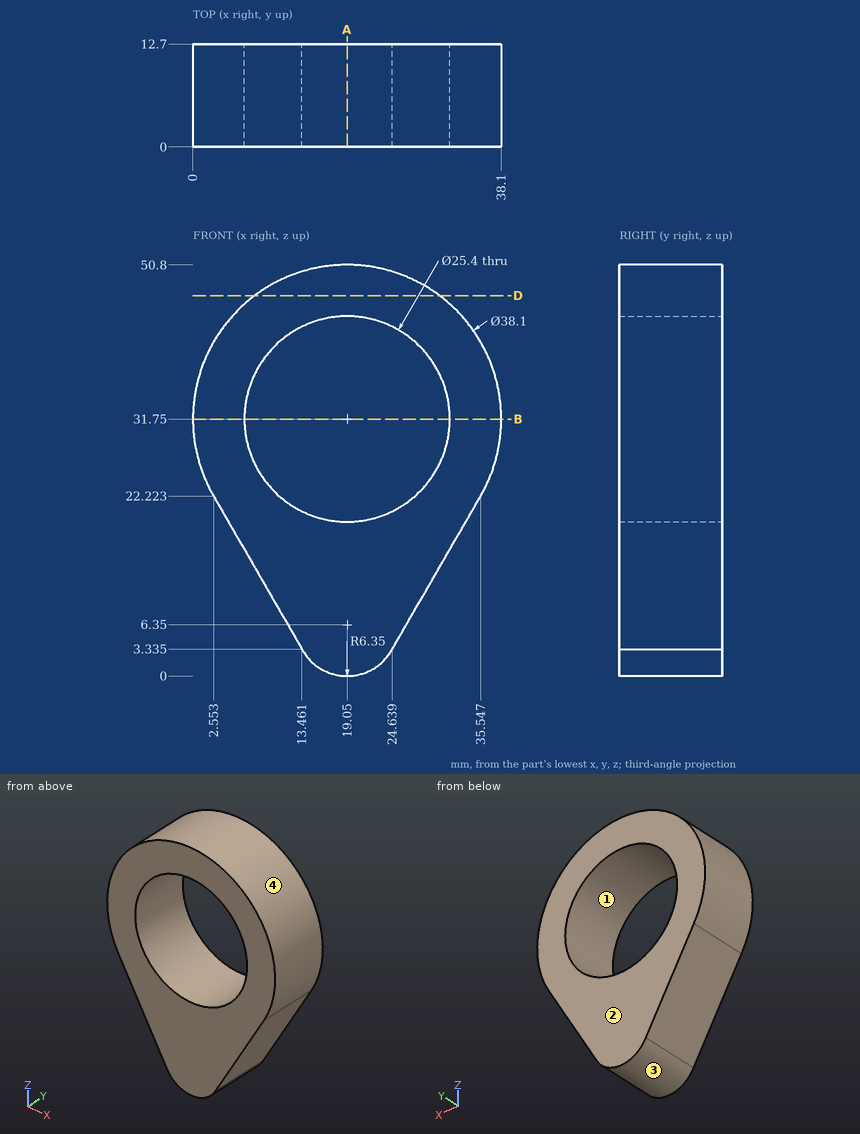
Print and shaded views of the part. All mm, measured from the part's lowest x, y and z. Coordinates: 2 decimals unless noted, no trailing zeros. Order: outer loops, then holes, each group sorted by start corner. A loop starts at its lowest first (then second) coordinate and runs counter-clockwise, first axis right, second up.
Item 1: Saw through at B-B on z = 31.75. List the corners of the cut face in (x, y).
Filled in:
outline: (0, 0) - (6.35, 0) - (6.35, 12.7) - (0, 12.7) - close; (31.75, 0) - (38.1, 0) - (38.1, 12.7) - (31.75, 12.7) - close
Item 2: Drop flat-ended pins along their axis: pin 1 Ø1 at (y, z) = (11, 38) entering from -X; pin 2 Ø5 at (x, y) = (22.5, 3.5) entering from +Z; pin 3 Ø5 at (x, y) = (5, 10) entering from +Z. Give the stop position or say it passes through.
Filled in:
pin 1: stops at x = 0.89
pin 2: stops at z = 50.78
pin 3: stops at z = 46.9
Item 3: Mould opens along Z. For the marked faces 1, 2, 3 and 4 say: released by +Z, released by -Z, zero draft, split by the parting line, or undercut.
Filled in:
face 1: undercut
face 2: zero draft
face 3: released by -Z
face 4: split by the parting line
Item 4: Drill centre lines: L1, parallel to Z at x = 19.05, y = 3.5; L2, parallel to X at y = 10.75, z = 28.5; L3, parallel to X at y = 9.5, z = 22 (1 decimal). Where is each one in solid material? Low to high.
Filled in:
L1: z = 0 to 19.05, 44.45 to 50.8
L2: x = 0.28 to 6.77, 31.33 to 37.82
L3: x = 2.7 to 10.9, 27.2 to 35.4
Item 5: Saw through at D-D on z = 47. List the corners of the cut face in (x, y), then the cut area to 3 significant figures.
Filled in:
outline: (7.63, 0) - (30.47, 0) - (30.47, 12.7) - (7.63, 12.7) - close
area: 290 mm2
Item 6: Saw through at A-A on x = 19.05. List the corners of the cut face in (y, z).
Filled in:
outline: (0, 0) - (12.7, 0) - (12.7, 19.05) - (0, 19.05) - close; (0, 44.45) - (12.7, 44.45) - (12.7, 50.8) - (0, 50.8) - close
